Read the model definition and answer for the solid it produces. Units are mm, in the model's axes. Face numbers are marked on the shaded views. Coordinates: 2 decimals unless noted, no trailing zeros. Loops run counter-clockwise (first coordinate to the right, second up) from the corner with the lowest first, then second, coordinate; pieces in that order, holes last.
Autodesk Inventor part; units mm, degrees
ref_plane "YZ Plane" through (0, 0, 0) normal (1, 0, 0) x (0, 1, 0)
ref_plane "XZ Plane" through (0, 0, 0) normal (0, 1, 0) x (-1, 0, 0)
ref_plane "XY Plane" through (0, 0, 0) normal (0, 0, 1) x (1, 0, 0)
sketch "Sketch1" plane through (0, 0, 0) normal (0, 1, 0) x (-1, 0, 0)
  circle A0 centre (0, 0) radius 10.5
  dimension "d0" = 21
extrude "Extrusion1" add sketch "Sketch1" along normal blind 70.8
sketch "Sketch2" plane through (0, 70.8, 0) normal (0, 1, 0) x (1, 0, 0)
  circle A0 centre (0, 0) radius 10.5
  line L0 (-10.5, 0) -> (-7, 0)
  circle A1 centre (0, 0) radius 7
  dimension "d3" = 3.5
extrude "Extrusion2" cut sketch "Sketch2" against normal blind 2 contours A1
sketch "Sketch3" plane through (0, 68.8, 0) normal (0, 1, 0) x (1, 0, 0)
  circle A0 centre (0, 0) radius 10.5
  line L0 (-10.5, 0) -> (-8.5, 0)
  circle A1 centre (0, 0) radius 8.5
  dimension "d6" = 2
extrude "Extrusion3" cut sketch "Sketch3" along normal blind 1.75 contours A1
sketch "Sketch4" plane through (0, 68.8, 0) normal (0, 1, 0) x (1, 0, 0)
  circle A0 centre (0, 0) radius 5.75
  dimension "d9" = 11.5
extrude "Extrusion4" add sketch "Sketch4" along normal blind 1.5
fillet "Fillet1" radius 1.5 1 edges at (-5.75, 70.3, 0)
sketch "Sketch5" plane through (0, 70.8, 0) normal (0, 1, 0) x (1, 0, 0)
  circle A0 centre (0, 0) radius 7
  circle A1 centre (0, 0) radius 7
  line L0 (0, 7) -> (0, 8.5)
  circle A2 centre (0, 0) radius 8.5
  circle A3 centre (0, 0) radius 4.25
  circle A4 centre (0, 0) radius 8.5
extrude "Extrusion5" cut sketch "Sketch5" against normal blind 0.05 contours A2
sketch "Sketch6" plane through (0, 0, 0) normal (0, -1, 0) x (1, 0, 0)
  circle A0 centre (0, 0) radius 10.5
  line L0 (0, 10.5) -> (0, 8.5)
  circle A1 centre (0, 0) radius 8.5
  circle A2 centre (0, 0) radius 8.5
  circle A3 centre (0, 0) radius 10.5
extrude "Extrusion6" cut sketch "Sketch6" against normal blind 0.05 contours A1
properties part number "baterka"
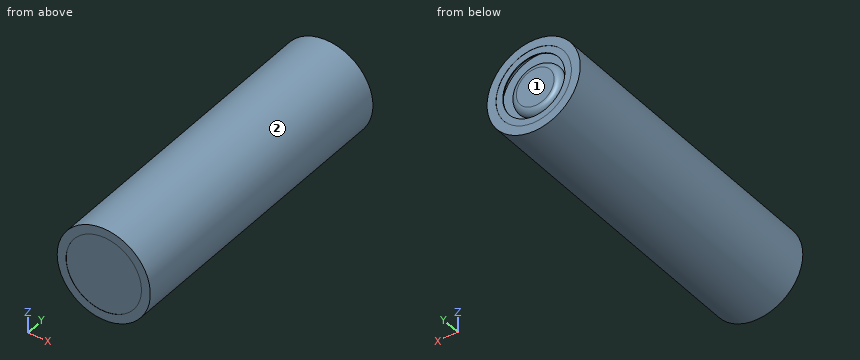
Item 1: Find the intervals of material crossed by line 1 along Y through (x, z) = (3.75, 6.5); line 2 along Y through (x, z) = (5, 4.5); line 3 along Y through (x, z) = (3, 0.75), in increasing order.
Numbers:
line 1: y = 0.05 to 68.8, 70.55 to 70.75
line 2: y = 0.05 to 68.8
line 3: y = 0.05 to 70.3
Item 2: Given pin 1 (8.5 mm diameter, centred on x = -2, z = 0.5, fed in from +Y); pin 2 (2 mm diameter, centred on y = 31, z = 0.5, fed in from +X); pin 3 (1 mm diameter, centred on x = 1.5, z = 3.5, fed in from -Y); pin 4 (10 mm diameter, centred on x = 6.5, y = 44.5, fed in from -Z), each flat-ended and moving along its own axis, determine where each tip first touches the part or whether it passes through.
Numbers:
pin 1: stops at y = 70.3
pin 2: stops at x = 10.5
pin 3: stops at y = 0.05
pin 4: stops at z = -10.39
Item 3: A cutting plane is placed at A-A on y = 6. Determine the outline of the cut face in (x, z).
Numbers:
outline: circle Ø21 at (0, 0)
Item 4: Determine the mould class of the marked faces 1 and 2 for opening direction X: released by +X, released by -X, zero draft, split by the parting line, or undercut.
Numbers:
face 1: undercut
face 2: split by the parting line
